Read the model definition and answer for the solid it produces. Units are mm, in the model's axes. Face numbers are marked on the shaded views. A direction names the side the tool comes from. Give positions to 0.01 mm unless a question says otherwise; leave off trailing zeros. Order: outer loops, then holes, each group sorted by start corner. A loop starts at its lowest first (then second) coordinate and runs counter-clockwise, first axis right, second up. Notation, with made-up numbers: M 22,-4.5 L 67,-4.5 A25 cw 67,19.5 Z; hole C 15,60.25 d10. An arc over 180 degrees is marked long. Write item = value, one per line. Start each with the question number.
Autodesk Inventor part; units mm, degrees
ref_plane "Plan de construction1" through (-13, -9.5, -10) normal (0, 0, -1) x (0, 1, 0)
ref_plane "YZ Plane" through (0, 0, 0) normal (1, 0, 0) x (0, 1, 0)
ref_plane "XZ Plane" through (0, 0, 0) normal (0, 1, 0) x (-1, 0, 0)
sketch "Esquisse1" plane through (0, 0, 0) normal (0, 0, 1) x (1, 0, 0)
  circle A0 centre (-3.5, 0) radius 2.5
  circle A1 centre (-3.5, 0) radius 2.5
  point P0 (0, 0)
ref_plane "Plan de construction1" through (-13, -9.5, -10) normal (0, 0, -1) x (0, 1, 0)
extrude "Extrusion1" add sketch "Esquisse1" against normal up to surface (10 mm away)
ref_plane "Plan de construction2" through (-3.5, 0, -9.5) normal (0, 0, -1) x (-1, 0, 0)
sketch "Esquisse2" plane through (-3.5, 0, -9.5) normal (0, 0, -1) x (-1, 0, 0)
  circle A0 centre (0, 0) radius 2.5
  circle A1 centre (0, 0) radius 2.2333
  point P0 (-3.5, 0)
extrude "Extrusion2" cut sketch "Esquisse2" along normal mid plane 0.5
sketch "Esquisxse8" plane through (-3.5, 0, 0) normal (0, 0, 1) x (1, 0, 0)
  circle A0 centre (-1.0139, -37.4629) radius 12
  circle A1 centre (-6.8791, -30.6366) radius 1.5
  circle A2 centre (-3.9931, -45.9556) radius 1.5
  circle A3 centre (7.8305, -35.7967) radius 1.5
  circle A4 centre (0, 0) radius 2.5
  arc A5 (6, 0) -> (-6, 0) centre (0, 0) ccw
  arc A6 (-12.7687, -35.0496) -> (10.3163, -33.5099) centre (-1.0139, -37.4629) ccw
  circle A7 centre (-3.9931, -45.9556) radius 1.5
  circle A8 centre (-6.8791, -30.6366) radius 1.5
  circle A9 centre (7.8305, -35.7967) radius 1.5
  line L0 (10.9482, -38.4158) -> (6, 0)
  line L1 (-6, 0) -> (-12.8221, -35.3258)
  point P0 (3.5, 0)
  dimension "d15" = 12
extrude "Extrusion6" add sketch "Esquisxse8" along normal blind 3 contours L0 A0 | A0 L1 A5 L0 picked at (-1.038, -37.5266)
sketch "Esquisse9" plane through (-3.5, 0, 3) normal (0, 0, 1) x (1, 0, 0)
  circle A0 centre (0, 0) radius 2.5
  circle A1 centre (0, 0) radius 2.5
  point P0 (3.5, 0)
extrude "Extrusion7" add sketch "Esquisse9" against normal blind 10
sketch "Esquisse11" plane through (-3.5, 0, 3) normal (0, 0, 1) x (1, 0, 0)
  circle A0 centre (-1.0139, -37.4629) radius 2.5
  point P0 (3.5, 0)
extrude "Extrusion8" cut sketch "Esquisse11" against normal blind 10
properties part number "bras_codeur"
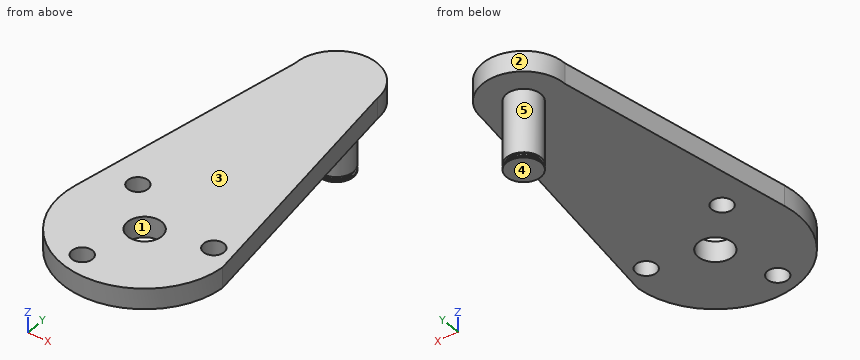
1) Find the intervals of material crossed by probe 1 along Z at (x, y) = (-8.5, -44.5); probe 2 along Y at (x, z) = (-5, 0.25); probe 3 along X at (y, z) = (-14.5, 2), in increasing order. Write a range as [from, to].
2) Find section C-C on x = -13.25. Determine the outline of the cut face in (y, z), plus the area to 3 significant figures.
3) Find section A-A on x = 4.5. Determine the outline of the cut face in (y, z), plus the area to 3 significant figures.
4) For the marked faces 4 and 5, determine the directions among +Z, -Z, +X, -X, +Y, -Y from which every point of the face is accessible in a straight line to the end or side of a thin tool.
5) For a pull along X with two mould halves and no side action, classify the marked faces 1, 2 and 3 as pulls with the +X half, pulls with the -X half, needs draft (parallel to the pull), parting line crosses it, or undercut.
6) Each of these flat-tipped pins is pushed along its axis until it touches: P1, Ø6, axis at x = -9.5, z = 1.5, coming from the +Y side; P2, Ø2.5, axis at x = 4.33, y = -35.8, coming from the -Z side; P3, Ø6, axis at x = -2, y = -37, coming from the -Z side; P4, Ø4, axis at y = -3.5, z = -8, coming from the +X side. Where does it stop, or does it pass through?
7) Find section D-D on z = -2. Determine the outline of the cut face in (x, y).
8) Find section B-B on z = 0.75. Determine the outline of the cut face in (x, y).
Numbers:
q1.probe_1 = [0, 3]
q1.probe_2 = [-49.45, -39.92], [-35.01, 5.81]
q1.probe_3 = [-12.3, 4.37]
q2.outline = M -45.69,0 L -19.42,0 L -19.42,3 L -45.69,3 Z
q2.area = 78.8 mm2
q3.outline = M -45.38,0 L -37.29,0 L -37.29,3 L -45.38,3 Z; M -34.31,0 L -15.53,0 L -15.53,3 L -34.31,3 Z
q3.area = 80.6 mm2
q4.face_4 = -Z, +X, -X, +Y, -Y
q4.face_5 = -Z
q5.face_1 = undercut
q5.face_2 = parting line crosses it
q5.face_3 = needs draft
q6.P1 = 5.2
q6.P2 = through
q6.P3 = 0
q6.P4 = -1.5
q7.outline = C -3.5,0 d5
q8.outline = M -16.27,-35.05 A12 ccw long 7.45,-38.42 L 2.5,0 A6 ccw -9.5,0 Z; hole C -10.38,-30.64 d3; hole C -7.49,-45.96 d3; hole C -4.51,-37.46 d5; hole C 4.33,-35.8 d3
